Geometry check sheet. Reference: drawing and pictorial views, mm from the part's lowest x, y, z. Coordinates: 2 decimals unless noted, no trailing zeros. Loops run counter-clockwise (first coordinate to the right, second up) from the corner with the lowest first, then second, coordinate; pieces in that order, holes last.
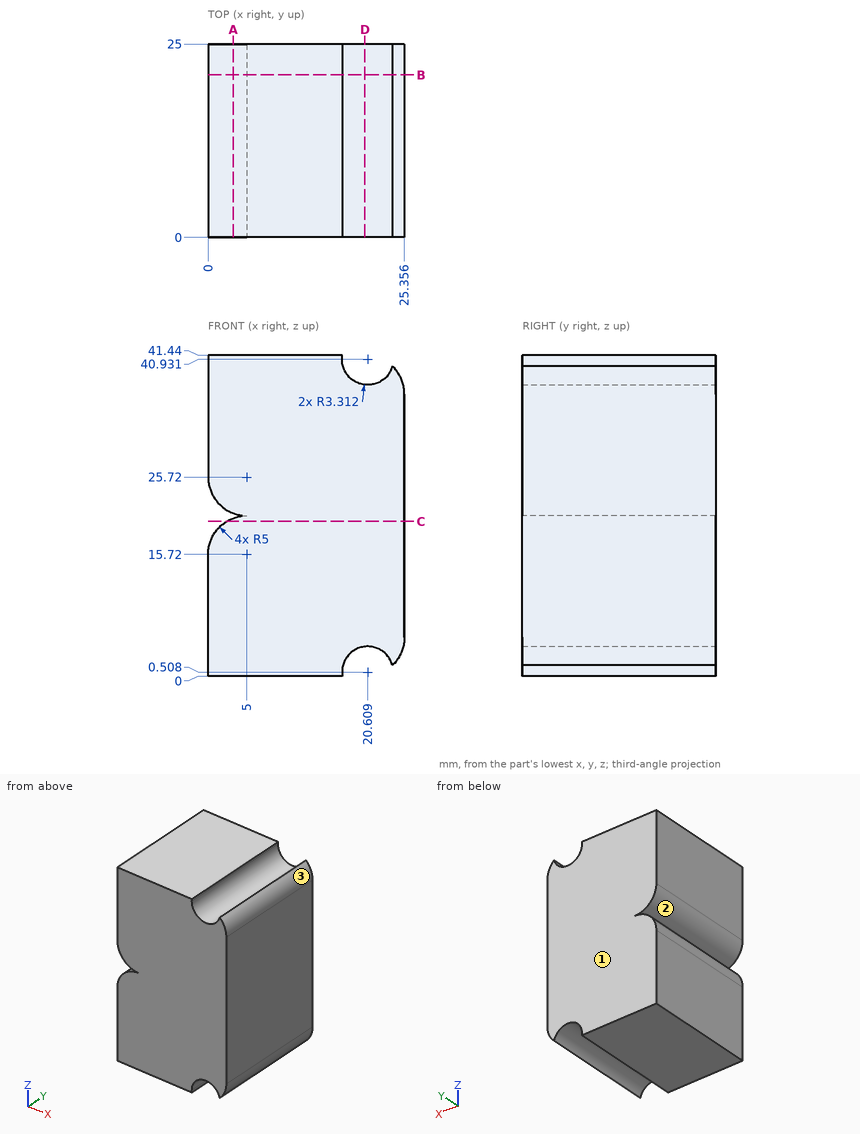
1) Material ranges on probe 1 along X at (y, z) = (16, 25); probe 2 along Z at (x, y) = (21.5, 23); probe 3 along X at (y, z) = (19.5, 37.5), recorded low to high.
Data:
probe 1: x = 0.05 to 25.36
probe 2: z = 3.7 to 37.74
probe 3: x = 0 to 25.24
2) Mould release check, pull along Z, two halves, no side actions. Record for the marked faces 1, 2 and 3: +Z half, -Z half, draft (parallel to the pull), parting line (faces both ways), or undercut.
Data:
face 1: draft
face 2: undercut
face 3: +Z half
3) Section check C-C on z = 20. Record the cut outline in (x, y) (1 decimal).
Data:
outline: (2.4, 0) - (25.4, 0) - (25.4, 25) - (2.4, 25) - close
4) Section check D-D on x = 20.25. Record the cut outline in (y, z), and give its area (3 significant figures).
Data:
outline: (0, 3.8) - (25, 3.8) - (25, 37.64) - (0, 37.64) - close
area: 846 mm2
5) Depth check by flat-ended pin: pin 1 (1.5 mm diameter, centred on x = 20, y = 20, fed in from +Z). Enter the tip coordinate at first touch or a pass-through.
Data:
pin 1: stops at z = 37.91
6) Section check B-B on y = 21. Record the cut outline in (x, z) (1 decimal), and give its area (3 significant figures).
Data:
outline: (0, 0) - (17.3, 0) arc R3.3 cw to (23.8, 1.4) arc R5 ccw to (25.4, 5) - (25.4, 36.4) arc R5 ccw to (23.8, 40.1) arc R3.3 cw to (17.3, 41.4) - (0, 41.4) - (0, 25.7) arc R5 ccw to (5, 20.7) arc R5 ccw to (0, 15.7) - close
area: 991 mm2
7) Section check A-A on x = 3.25. Record the cut outline in (y, z).
Data:
outline: (0, 0) - (25, 0) - (25, 20.4) - (0, 20.4) - close; (0, 21.04) - (25, 21.04) - (25, 41.44) - (0, 41.44) - close
